Check sheet for the modelled part. Datum: model origin and axes. Units: mm. A direction names the side the tool comes from. Round coordinates to 2 decimals unless told otherwise and drop trailing zeros. Write each loop counter-clockwise with the first axis right and the second up, starting at its lowest first coordinate (ties: lowest second). Pieces come first, ordered by that corner, then holes.
Item 1: Set-up check for faces 1 (the flat face through (0, 17.05, 8)), 2 (the flat face through (-17, -15, 16.3)), 3 (the flat face through (-18.69, 0, 11)), 4 (the flat face through (-6.386, -18, 14)), 5 (the cylindrical face through (-17.88, 0.05, 19.44)): record each of +Z, -Z, +X, -X, +Y, -Y from which the full face is reachable in a straight line by a thin tool's end or side.
Item 2: Section check A-A, the plane y = 0. Record the cut outline in (x, z), plus the area to 3 significant figures.
Item 3: Section check C-C, the plane x = -9.5. Record the cut outline in (y, z), plus the area to 3 significant figures.
Item 4: Section check D-D, the plane y = -16. Record the cut outline in (x, z).
Item 5: Depth check by flat-ended pin: pin 1 (1.7 mm diameter, centred on x = -16.5, y = -14.5, fed in from +Z); pin 2 (0.8 mm diameter, centred on y = -17.5, z = 14.5, fed in from +X); pin 3 (1.8 mm diameter, centred on x = -3, y = -17.5, fed in from +Z); pin 4 (5 mm diameter, centred on x = 14.5, y = -5.5, fed in from -Z). Enter the tip coordinate at first touch or a pass-through.
Item 6: Section check B-B, the plane z = 7.75. Record the cut outline in (x, y), plus the area to 3 significant figures.
Item 7: Release check for a two-part mould opening along Z. For faces 6 (the cylindrical face through (-11.98, -17.89, 15.7)), 7 (the cylindrical face through (17.86, 12.2, 2.97)), 8 (the cylindrical face through (-17.9, -0.2, 9.9)), 9 (the flat face through (17.05, 0, 6)) record: pulls with the +Z half, pulls with the -Z half, needs draft (parallel to the pull), parting line crosses it, or undercut.
Item 8: Material ranges on line 1 along Y through (x, z) = (1.5, 10); line 2 along X through (y, z) = (15.5, 5), recorded low to high.
Autodesk Inventor part; units mm, degrees
ref_plane "РабПлоскость1" through (-16.75, -17.4, 16.3) normal (0, 0, 1) x (1, 0, 0)
ref_plane "РабПлоскость2" through (19.19, -20.45, 0) normal (-1, 0, 0) x (0, 0, 1)
ref_plane "YZ Plane" through (0, 0, 0) normal (1, 0, 0) x (0, 1, 0)
ref_plane "РабПлоскость1" through (-16.75, -17.4, 16.3) normal (0, 0, 1) x (1, 0, 0)
sketch "Эскиз1" plane through (0, 0, 0) normal (0, 0, 1) x (1, 0, 0)
  line L0 (-18.1779, 4.2816) -> (-18.69, 4.2816)
  line L1 (-18.69, 4.2816) -> (-18.69, -13.75)
  arc A0 (-18.69, -13.75) -> (-13.75, -18.69) centre (-13.75, -13.75) ccw
  line L2 (-13.75, -18.69) -> (13.75, -18.69)
  arc A1 (13.75, -18.69) -> (18.69, -13.75) centre (13.75, -13.75) ccw
  line L3 (18.69, -13.75) -> (18.69, 13.75)
  arc A2 (18.69, 13.75) -> (13.75, 18.69) centre (13.75, 13.75) ccw
  line L4 (13.75, 18.69) -> (-13.75, 18.69)
  arc A3 (-13.75, 18.69) -> (-18.69, 13.75) centre (-13.75, 13.75) ccw
  line L5 (-18.69, 13.75) -> (-18.69, 9.7184)
  line L6 (-18.69, 9.7184) -> (-18.1779, 9.7184)
  line L7 (-18.1779, 13.75) -> (-18.1779, 9.7184)
  arc A4 (-13.75, 18.1779) -> (-18.1779, 13.75) centre (-13.75, 13.75) ccw
  line L8 (13.75, 18.1779) -> (-13.75, 18.1779)
  arc A5 (18.1779, 13.75) -> (13.75, 18.1779) centre (13.75, 13.75) ccw
  line L9 (18.1779, -13.75) -> (18.1779, 13.75)
  arc A6 (13.75, -18.1779) -> (18.1779, -13.75) centre (13.75, -13.75) ccw
  line L10 (-13.75, -18.1779) -> (13.75, -18.1779)
  arc A7 (-18.1779, -13.75) -> (-13.75, -18.1779) centre (-13.75, -13.75) ccw
  line L11 (-18.1779, 4.2816) -> (-18.1779, -13.75)
  line L12 (-18.1779, 4.2816) -> (-18.69, 4.2816)
  line L13 (-18.69, 4.2816) -> (-18.69, 9.7184)
  line L14 (-18.69, 9.7184) -> (-18.1779, 9.7184)
  line L15 (-18.1779, 9.7184) -> (-18.1779, 4.2816)
  line L16 (-13.75, 16.45) -> (10.2, 16.45)
  arc A8 (-13.75, 16.45) -> (-16.75, 13.45) centre (-13.75, 13.45) ccw
  line L17 (-16.75, -10.2) -> (-16.75, 13.45)
  arc A9 (-16.75, -10.2) -> (-15.75, -11.2) centre (-15.75, -10.2) ccw
  line L18 (-14.1, -11.2) -> (-15.75, -11.2)
  arc A10 (-11.2, -14.1) -> (-14.1, -11.2) centre (-14.1, -14.1) ccw
  line L19 (-11.2, -14.1) -> (-11.2, -15.75)
  arc A11 (-11.2, -15.75) -> (-10.2, -16.75) centre (-10.2, -15.75) ccw
  line L20 (-6.3858, -16.75) -> (-10.2, -16.75)
  arc A12 (-5.9929, -17.075) -> (-6.3858, -16.75) centre (-6.3858, -17.15) ccw
  arc A13 (-5.9929, -17.075) -> (-5.6, -17.4) centre (-5.6, -17) ccw
  line L21 (-5.6, -17.4) -> (5.6, -17.4)
  arc A14 (5.6, -17.4) -> (5.9929, -17.075) centre (5.6, -17) ccw
  arc A15 (6.3858, -16.75) -> (5.9929, -17.075) centre (6.3858, -17.15) ccw
  line L22 (12.1982, -16.75) -> (6.3858, -16.75)
  arc A16 (12.1982, -16.75) -> (13.1981, -15.7356) centre (12.1982, -15.75) ccw
  arc A17 (15.7351, -13.198) -> (13.1981, -15.7356) centre (15.6978, -15.6978) ccw
  arc A18 (15.7351, -13.198) -> (16.75, -12.1982) centre (15.75, -12.1982) ccw
  line L23 (16.75, -12.1982) -> (16.75, 10.2)
  arc A19 (16.75, 10.2) -> (15.75, 11.2) centre (15.75, 10.2) ccw
  line L24 (14.1, 11.2) -> (15.75, 11.2)
  arc A20 (11.2, 14.1) -> (14.1, 11.2) centre (14.1, 14.1) ccw
  line L25 (11.2, 15.45) -> (11.2, 14.1)
  arc A21 (11.2, 15.45) -> (10.2, 16.45) centre (10.2, 15.45) ccw
  circle A22 centre (7, 14.5) radius 0.95
  circle A23 centre (0, 14.6) radius 0.75
  circle A24 centre (-7.5, -13.8) radius 0.95
  circle A25 centre (-14.9, 2) radius 0.75
  circle A26 centre (8.272, -2.7758) radius 0.5
  circle A27 centre (8.6932, -0.0132) radius 0.5
  circle A28 centre (8.2597, 2.7621) radius 0.5
  circle A29 centre (-2.2984, 14.2551) radius 0.5
  circle A30 centre (-4.5412, 14.2552) radius 0.5
  circle A31 centre (13.75, -13.75) radius 3.5
  circle A32 centre (-13.75, -13.75) radius 3.5
  circle A33 centre (13.75, 13.75) radius 3.5
  circle A34 centre (-13.75, 13.75) radius 3.5
  line L26 (-17.25, 13.75) -> (-17.25, -13.75)
  line L27 (-13.75, -17.25) -> (13.75, -17.25)
  line L28 (17.25, -13.75) -> (17.25, 13.75)
  line L29 (13.75, 17.25) -> (-13.75, 17.25)
  arc A35 (13.75, -17.25) -> (17.25, -13.75) centre (13.75, -13.75) ccw
  arc A36 (-17.25, -13.75) -> (-13.75, -17.25) centre (-13.75, -13.75) ccw
  arc A37 (-13.75, 17.25) -> (-17.25, 13.75) centre (-13.75, 13.75) ccw
  arc A38 (17.25, 13.75) -> (13.75, 17.25) centre (13.75, 13.75) ccw
  line L30 (-13.75, 17.05) -> (13.75, 17.05)
  arc A39 (17.05, 13.75) -> (13.75, 17.05) centre (13.75, 13.75) ccw
  line L31 (17.05, 13.75) -> (17.05, -13.75)
  arc A40 (13.75, -17.05) -> (17.05, -13.75) centre (13.75, -13.75) ccw
  line L32 (13.75, -17.05) -> (-13.75, -17.05)
  arc A41 (-17.05, -13.75) -> (-13.75, -17.05) centre (-13.75, -13.75) ccw
  line L33 (-17.05, -13.75) -> (-17.05, 13.75)
  arc A42 (-13.75, 17.05) -> (-17.05, 13.75) centre (-13.75, 13.75) ccw
  line L34 (6.3858, -18.69) -> (-6.3858, -18.69)
  line L35 (-6.3858, -18.69) -> (-6.3858, -14.69)
  line L36 (-6.3858, -14.69) -> (6.3858, -14.69)
  line L37 (6.3858, -14.69) -> (6.3858, -18.69)
  point P0 (0, 0)
  point P1 (12.5838, -17.05)
  point P2 (5.9122, -17.25)
  point P3 (5.9985, -17.05)
  point P4 (-6.3858, -17.05)
  point P5 (6.3858, -17.05)
  point P6 (-6.3858, -18.69)
  dimension "d0" = 7
  dimension "d2" = 7
  dimension "d3" = 7
  dimension "d4" = 7
  dimension "d5" = 0.2
  dimension "d8" = 4
extrude "Выдавливание1" add sketch "Эскиз1" along normal up to surface (16.3 mm away) contours L11 A7 L10 L35 L2 A0 L1 L0 | L15 L7 A4 L8 A5 L9 A6 L10 L37 L27 A31 L28 A33 L29 A34 L26 A32 L35 A7 L11 | L0 L13 L6 L15 | L6 L5 A3 L4 A2 L3 A1 L2 L37 L10 A6 L9 A5 L8 A4 L7 | L27 A32 L32 L35 | L37 L32 A31 L27 | A32 L33 A41 L32 | A31 L32 A40 L31 | L26 A34 L33 A32 | A31 L31 A33 L28 | A34 L30 A42 L33 | A33 L31 A39 L30 | L29 A33 L30 A34
sketch "Эскиз2" plane through (0, 0, 0) normal (0, 0, -1) x (-1, 0, 0)
  line L0 (6.3858, -18.69) -> (6.3858, -17.05)
  line L1 (-6.3858, -17.05) -> (-6.3858, -18.69)
  line L2 (6.3858, -18.69) -> (-6.3858, -18.69)
  line L3 (-6.3858, -18.69) -> (-6.3858, -17.05)
  line L4 (-6.3858, -17.05) -> (6.3858, -17.05)
  line L5 (6.3858, -17.05) -> (6.3858, -18.69)
  point P0 (0, 0)
extrude "Выдавливание2" add sketch "Эскиз2" against normal blind 11
sketch "Эскиз3" plane through (-18.69, -13.75, 0) normal (-1, 0, 0) x (0, 0, 1)
  circle A0 centre (-8.4, 13.75) radius 18.69
  line L0 (0, 13.75) -> (16.3, 13.75)
  line L1 (16.3, 27.5) -> (16.3, 0)
  circle A1 centre (-8.4, 13.75) radius 14.8
  line L2 (0, 13.75) -> (16.3, 13.75)
  line L3 (0, 0) -> (0, 27.5)
  circle A2 centre (8.15, 13.75) radius 1.75
  circle A3 centre (-8.4, 13.75) radius 18.3
  circle A4 centre (4.0904, 24.6078) radius 1.75
  circle A5 centre (4.0904, 2.8922) radius 1.75
  line L4 (-8.4, 13.75) -> (22.7381, 2.4167)
  line L5 (-8.4, 13.75) -> (22.7381, 25.0833)
  line L6 (4.0904, 2.8922) -> (-8.4, 13.75)
  line L7 (-8.4, 13.75) -> (4.0904, 24.6078)
  circle A6 centre (7.5861, 18.0335) radius 1.75
  circle A7 centre (7.5861, 9.4665) radius 1.75
  line L8 (-8.4, 13.75) -> (7.5861, 18.0335)
  line L9 (7.5861, 9.4665) -> (-8.4, 13.75)
  point P0 (5.4112, 25.7559)
  point P1 (2.7697, 23.4597)
  point P2 (2.7697, 4.0403)
  point P3 (5.4112, 1.7441)
  dimension "d12" = 3.5
  dimension "d13" = 3.5
  dimension "d14" = 3.5
  dimension "d26" = 30
  dimension "d27" = 15
  dimension "d28" = 26
  dimension "d29" = 26
extrude "Выдавливание3" cut sketch "Эскиз3" against normal blind 40 contours A2 L0 | L0 A2 | A3 A7 A1 A2 | A2 A1 A6 A3 | L5 A6 A1 A4 A3 | A3 A6 L5 | L4 A7 A3 | A3 A5 A1 L4 A7 | A6 L5 | A7 L4 | A4 | L5 A6 | A5 | A7 L4 | A1 L5 A6 | A7 L4 A1
sketch "Эскиз5" plane through (-18.69, -13.75, 16.3) normal (-1, 0, 0) x (0, 0, 1)
  circle A0 centre (4.2399, 13.75) radius 1.1
  circle A1 centre (4.2399, 13.75) radius 1.8
  line L0 (5.8801, 13.0086) -> (0, 0)
  line L1 (0, 27.5) -> (0, 0)
  line L2 (5.8801, 14.4914) -> (0, 27.5)
  point P0 (-16.3, 13.75)
  dimension "d23" = 3.6
extrude "Выдавливание5" add sketch "Эскиз5" against normal up to surface (1.64 mm away)
sketch "Эскиз6" plane through (-18.69, -13.75, 0) normal (-1, 0, 0) x (0, 0, 1)
  circle A0 centre (-8.4, 13.75) radius 30.7399
  line L0 (0, -3.3) -> (16.3, -3.3)
  line L1 (0, 30.8) -> (16.3, 30.8)
  line L2 (16.3, -3.3) -> (16.3, 0)
  circle A1 centre (-8.4, 13.75) radius 30.0132
  circle A2 centre (-8.4, 13.75) radius 32.0132
  line L3 (16.3, -3.3) -> (18.6951, -3.3)
  line L4 (11, -4.94) -> (16.3, -4.94)
  line L5 (15.0835, -4.94) -> (17.5909, -4.94)
  line L6 (0, 30.8) -> (16.3, 30.8)
  line L7 (16.3, 30.8) -> (18.6951, 30.8)
  line L8 (0, 32.44) -> (16.3, 32.44)
  line L9 (15.0835, 32.44) -> (17.5909, 32.44)
  point P0 (0, 13.75)
  point P1 (16.3, 30.8)
  dimension "d30" = 2
ref_plane "РабПлоскость2" through (19.19, -20.45, 0) normal (-1, 0, 0) x (0, 0, 1)
extrude "Выдавливание6" cut sketch "Эскиз6" against normal blind 40 contours L7 A1 L8 A0 | A0 L8 L9 A2 L7 | L3 A2 L5 L4 A0 | A0 L4 A1 L3
equation "\"d27\" = 0.5 * d26"
properties part number "lidar_base"
Values found:
1. face 1: +Z, -Z
1. face 2: +Z, +X, -X, -Y
1. face 3: +Z, -Z, -X, +Y, -Y
1. face 4: +Z, -Y
1. face 5: +X, -X
2. outline: (-18.69, 0) - (-17.05, 0) - (-17.05, 6.4) - (-18.69, 6.4) - close; (-18.69, 9.9) - (-17.05, 9.9) - (-17.05, 19.44) - (-18.69, 19.44) - close; (-18.69, 21.64) - (-17.05, 21.64) - (-17.05, 22.34) - (-18.69, 22.34) - close; (17.05, 0) - (18.69, 0) - (18.69, 6.4) - (17.05, 6.4) - close; (17.05, 9.9) - (18.69, 9.9) - (18.69, 16.3) - (17.05, 16.3) - close
2. area: 48.3 mm2
3. outline: (-18.69, 0) - (-17.05, 0) - (-17.05, 16.3) arc R30.01 ccw to (-18.69, 15.08) - close; (17.05, 0) - (18.69, 0) - (18.69, 15.08) arc R30.01 ccw to (17.05, 16.3) - close
3. area: 51.5 mm2
4. outline: (-18.15, 0) - (-16.16, 0) - (-16.16, 16.3) - (-18.15, 16.3) - close; (16.16, 0) - (18.15, 0) - (18.15, 16.3) - (16.16, 16.3) - close
5. pin 1: stops at z = 16.3
5. pin 2: stops at x = 17.38
5. pin 3: stops at z = 11
5. pin 4: passes through
6. outline: (-18.69, -13.75) arc R4.94 ccw to (-13.75, -18.69) - (13.75, -18.69) arc R4.94 ccw to (18.69, -13.75) - (18.69, -8.61) - (17.05, -8.61) - (17.05, -13.75) arc R3.3 cw to (13.75, -17.05) - (-13.75, -17.05) arc R3.3 cw to (-17.05, -13.75) - (-17.05, -8.61) - (-18.69, -8.61) - close; (-18.69, 8.61) - (-17.05, 8.61) - (-17.05, 13.75) arc R3.3 cw to (-13.75, 17.05) - (13.75, 17.05) arc R3.3 cw to (17.05, 13.75) - (17.05, 8.61) - (18.69, 8.61) - (18.69, 13.75) arc R4.94 ccw to (13.75, 18.69) - (-13.75, 18.69) arc R4.94 ccw to (-18.69, 13.75) - close
6. area: 166 mm2
7. face 6: pulls with the +Z half
7. face 7: undercut
7. face 8: undercut
7. face 9: needs draft
8. line 1: y = -18.69 to -17.05, 17.05 to 18.69
8. line 2: x = -18.37 to -16.55, 16.55 to 18.37
